Here's the drawing with two shaded views (mm, measured from the low corner). I have some questions. A direction names the side the tool comes from. Coordinates: 2 decimals unless noted, no trailing zeros. Write each loop counter-clockwise with the first axis right and the second up, starting at its lowest first coordinate (ties: lowest second). Pieces come first, ordered by that corner, then holes.
Item 1: For P1, Ø6.5, axis at y = 7.5, z = 5, coming from the +X side; P2, Ø2, axis at x = 10, y = 11, coming from the -Z side; P3, Ø5, axis at x = 8.5, y = 11, coming from the +Z side, each with a flat end and sliding along its axis, tell me the tip position at first contact or that it passes through.
Item 2: Thinking about a two-plate mould opening in X: for the marked faces 1, 2, 3 and 4, which applies, +X half, -X half, draft (parallel to the pull), parting line (faces both ways), or undercut?
Item 3: Which directions (+Z, -Z, +X, -X, +Y, -Y) give clear straight access to the entire face, cutting with the end or side of a thin tool? Please do the marked faces 5 and 6.
Item 4: If I drill on probe 1 along Y at (x, z) = (5.6, 5); probe 2 along Y at (x, z) = (2.4, 5); probe 3 along Z at (x, y) = (2.5, 7.75), over which ranges is the centre line in solid material (lowest first)?
Item 5: I want a section at B-B on z = 5. Please give me the cut outline in (x, y).
Item 6: I want a section at C-C on z = 22.5. Please give me the cut outline in (x, y).
Item 7: I want a section at A-A on y = 7.5. Please give me the cut outline in (x, z), then the cut area to 3 significant figures.
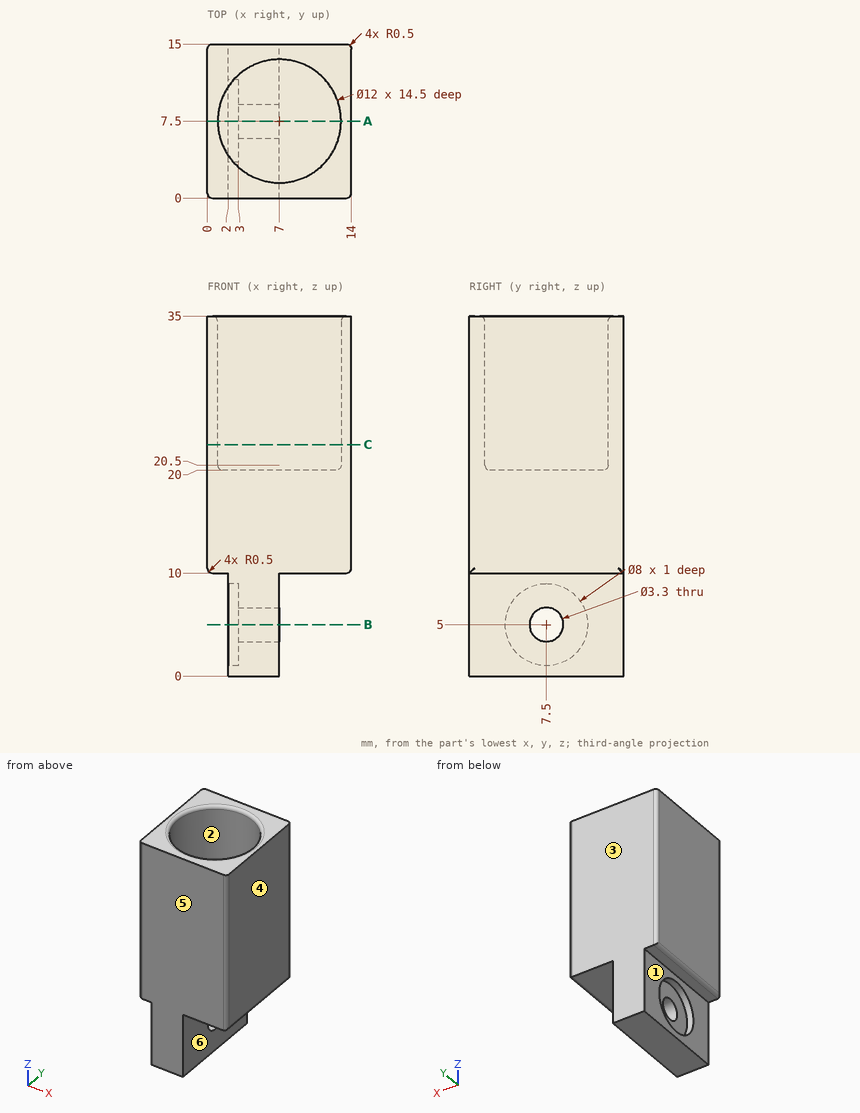
Response values:
1. P1: stops at x = 7
1. P2: stops at z = 10
1. P3: stops at z = 34.96
2. face 1: -X half
2. face 2: undercut
2. face 3: draft
2. face 4: +X half
3. face 5: +Z, -Z, +X, -X, -Y
3. face 6: -Z, +X, +Y, -Y
4. probe 1: y = 0 to 5.85, 9.15 to 15
4. probe 2: y = 0 to 3.5, 11.5 to 15
4. probe 3: z = 0 to 1.01, 8.99 to 20
5. outline: (2, 0) - (7, 0) - (7, 5.85) - (3, 5.85) - (3, 3.5) - (2, 3.5) - close; (2, 11.5) - (3, 11.5) - (3, 9.15) - (7, 9.15) - (7, 15) - (2, 15) - close
6. outline: (0, 0.5) arc R0.5 ccw to (0.5, 0) - (13.5, 0) arc R0.5 ccw to (14, 0.5) - (14, 14.5) arc R0.5 ccw to (13.5, 15) - (0.5, 15) arc R0.5 ccw to (0, 14.5) - close; hole circle Ø12 at (7, 7.5)
7. outline: (0, 10.5) arc R0.5 ccw to (0.5, 10) - (2, 10) - (2, 9) - (3, 9) - (3, 6.65) - (7, 6.65) - (7, 10) - (13.5, 10) arc R0.5 ccw to (14, 10.5) - (14, 35) - (13.5, 35) arc R0.5 ccw to (13, 34.5) - (13, 20.5) arc R0.5 cw to (12.5, 20) - (1.5, 20) arc R0.5 cw to (1, 20.5) - (1, 34.5) arc R0.5 ccw to (0.5, 35) - (0, 35) - close; (2, 0) - (7, 0) - (7, 3.35) - (3, 3.35) - (3, 1) - (2, 1) - close
7. area: 199 mm2
